Check sheet for the modelled part. Datum: model origin and axes. Units: mm. Face numbers are marked on the shaded views. A direction names the side the tool comes from. Round coordinates to 2 decimals unless told otherwise and drop trailing zeros. Loops run counter-clockwise (first coordinate to the right, second up) from the corner with the lowest first, then second, coordinate; pieces in that order, holes last. Notation, with made-up numbers: (-32, -26) - (1, -26) arc R15 ccw to (1, 0) - close; hole circle Ø11 at (-37, 84). An arc over 180 degrees is marked (long way). Answer in a Markdown table with one row per item. Add a question column.
(1) Access from +Z, -Z, +X, -X, +Y, -Y to the whole of each face (thin tool, end or side, straight path). Record for the marked faces 4, 5, 6, 7 and 8.
(2) Cross-section at C-C on y = -9.5. Enter the section's corners in (x, z), then the cut area to 3 significant figures.
(3) Mould release check, pull along X, two halves, no side actions. Record for the marked faces 1, 2 and 3: +X half, -X half, draft (parallel to the pull), parting line (faces both ways), or undercut.
(4) Thickness scan on line 1 along X through (y, z) = (-24.5, 20); line 2 along X through (y, z) = (-19, 85.5); line 3 along Z through (x, y) = (-46, -16). Record the ranges inside material, lowest first.
(5) Cross-section at D-D on x = -34. Enter the section's corners in (y, z).
(6) Cross-section at A-A on z = 18. Enter the section's corners in (x, y).
(7) Cross-section at B-B on z = 29.5. Enter the section's corners in (x, y).
(8) Gauge pin test, flat ends, axial feed: pin 1 (1 mm diameter, centred on x = 29.5, y = -35.5, fed in from -Z); pin 2 (1 mm diameter, centred on y = -40, z = 86.5, fed in from -X); pin 3 (7.5 mm diameter, centred on x = 16.5, y = -37, fed in from +Z). Record the tip position at first contact, or that the pin passes through.
from build123d import *

# Parameters (mm, degrees)
F0_W     = 101.6
F0_H     = 88.9
F1_DEPTH = 63.5
F2_W     = 25.4
F2_H     = 25.4
F3_DEPTH = 63.5
F4_W     = 25.4
F4_H     = 25.4
F5_DEPTH = 63.5
F6_W     = 76.2
F6_H     = 12.7
F7_DEPTH = 63.5
F8_W     = 35.461226
F8_H     = 18.227942
F9_DEPTH = 25.4


with BuildPart() as f1:
    # F0 (on Front) → F1 (new body)
    with BuildSketch(Plane.XZ):
        with Locations((-23.928717, 52.601962)):
            Rectangle(F0_W, F0_H)
    extrude(amount=F1_DEPTH)

    # F2 (on face) → F3 (cut)
    with BuildSketch(Plane.XZ.offset(63.5)):
        with Locations((-62.028717, 84.351962)):
            Rectangle(F2_W, F2_H)
    extrude(amount=-F3_DEPTH, mode=Mode.SUBTRACT)

    # F4 (on face) → F5 (cut)
    with BuildSketch(Plane.XZ.offset(63.5)):
        with Locations((14.171283, 84.351962)):
            Rectangle(F4_W, F4_H)
    extrude(amount=-F5_DEPTH, mode=Mode.SUBTRACT)

    # F6 (on face) → F7 (cut)
    with BuildSketch(Plane.XZ.offset(63.5)):
        with Locations((-23.928717, 14.501962)):
            Rectangle(F6_W, F6_H)
    extrude(amount=-F7_DEPTH, mode=Mode.SUBTRACT)

    # F8 (on face) → F9 (join)
    with BuildSketch(Plane.YZ.offset(26.871283)):
        with Locations((-30.654847, 32.522842)):
            Rectangle(F8_W, F8_H)
    extrude(amount=F9_DEPTH)


solid = f1.part
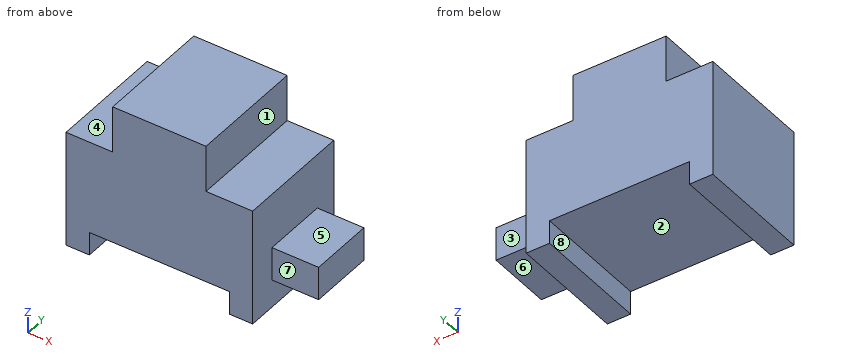
Answers:
| question | item | result |
|---|---|---|
| 1 | face 4 | +Z, -X, +Y, -Y |
| 1 | face 5 | +Z, +X, +Y, -Y |
| 1 | face 6 | -Z, +X, +Y, -Y |
| 1 | face 7 | +Z, -Z, +X, -Y |
| 1 | face 8 | -Z, +Y, -Y |
| 2 | outline | (-74.73, 8.15) - (-62.03, 8.15) - (-62.03, 20.85) - (14.17, 20.85) - (14.17, 8.15) - (26.87, 8.15) - (26.87, 71.65) - (1.47, 71.65) - (1.47, 97.05) - (-49.33, 97.05) - (-49.33, 71.65) - (-74.73, 71.65) - close |
| 2 | area | 6,770 mm^2 |
| 3 | face 1 | +X half |
| 3 | face 2 | undercut |
| 3 | face 3 | draft |
| 4 | line 1 | x = -74.73 to -62.03, 14.17 to 26.87 |
| 4 | line 2 | x = -49.33 to 1.47 |
| 4 | line 3 | z = 20.85 to 97.05 |
| 5 | outline | (-63.5, 20.85) - (0, 20.85) - (0, 97.05) - (-63.5, 97.05) - close |
| 6 | outline | (-74.73, -63.5) - (-62.03, -63.5) - (-62.03, 0) - (-74.73, 0) - close; (14.17, -63.5) - (26.87, -63.5) - (26.87, 0) - (14.17, 0) - close |
| 7 | outline | (-74.73, -63.5) - (26.87, -63.5) - (26.87, -48.39) - (52.27, -48.39) - (52.27, -12.92) - (26.87, -12.92) - (26.87, 0) - (-74.73, 0) - close |
| 8 | pin 1 | stops at z = 23.41 |
| 8 | pin 2 | stops at x = -49.33 |
| 8 | pin 3 | stops at z = 71.65 |
